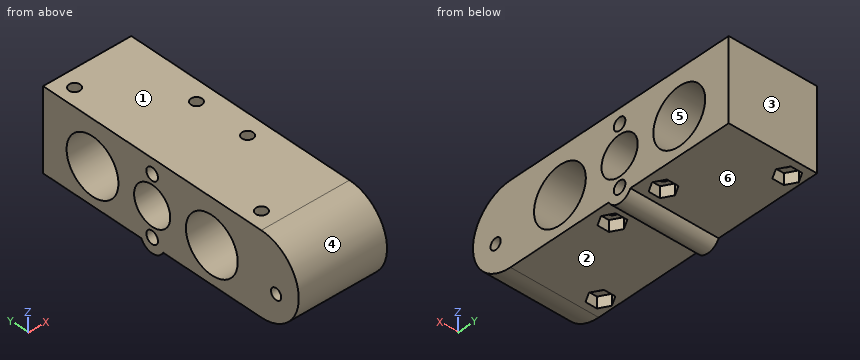
```python
from build123d import *

# Parameters (mm, degrees)
SKETCH035_R          = 7.6
SKETCH035_R_2        = 1.5
PAD011_DEPTH         = 24
SKETCH034_R          = 5.3
SKETCH034_R_2        = 1.7
POCKET021_DEPTH      = 24.001
SKETCH036_R          = 1.5
POCKET022_DEPTH      = 22.001
POCKET022_DEPTH_BACK = 2.001
POCKET023_DEPTH      = 3


with BuildPart() as part:
    # Sketch035 → Pad011 (new body)
    with BuildSketch(Plane.YZ):
        with BuildLine():
            Line((-32, 12), (32, 12))
            Line((32, 12), (32, -10))
            Line((3.1622776602, -10), (32, -10))
            ThreePointArc((-3.1622776602, -10), (0, -12), (3.1622776602, -10))
            Line((-32, -10), (-3.1622776602, -10))
            ThreePointArc((-32, 12), (-43, 1), (-32, -10))
        make_face()
        with Locations((17.5, 0)):
            Circle(SKETCH035_R, mode=Mode.SUBTRACT)
        with Locations((-17.5, 0)):
            Circle(SKETCH035_R, mode=Mode.SUBTRACT)
        with Locations((-36.35, -1.62)):
            Circle(SKETCH035_R_2, mode=Mode.SUBTRACT)
    extrude(amount=PAD011_DEPTH)

    # Sketch034 → Pocket021 (cut, through all)
    with BuildSketch(Plane(origin=(0, 0, 0), x_dir=(0, 0.7071067812, 0.7071067812), z_dir=(1, 0, 0))):
        Circle(SKETCH034_R)
        with Locations((5.65, 5.65)):
            Circle(SKETCH034_R_2)
        with Locations((-5.65, -5.65)):
            Circle(SKETCH034_R_2)
    extrude(amount=POCKET021_DEPTH, mode=Mode.SUBTRACT)

    # Sketch036 (on DatumPlane) → Pocket022 (cut, two sides)
    with BuildSketch(Plane.YX.offset(10)) as pocket022_sk:
        with Locations((-7.5, 19)):
            Circle(SKETCH036_R)
        with Locations((7.5, 19)):
            Circle(SKETCH036_R)
        with Locations((27.4, 4.3)):
            Circle(SKETCH036_R)
        with Locations((-27.4, 4.3)):
            Circle(SKETCH036_R)
    extrude(amount=-POCKET022_DEPTH, mode=Mode.SUBTRACT)
    extrude(pocket022_sk.sketch, amount=POCKET022_DEPTH_BACK, mode=Mode.SUBTRACT)

    # Sketch037 (on DatumPlane) → Pocket023 (cut)
    with BuildSketch(Plane.YX.offset(10)):
        Polygon((-24.7, 5.3588457268), (-27.4, 6.9176914536), (-30.1, 5.3588457268), (-30.1, 2.2411542732), (-27.4, 0.6823085464), (-24.7, 2.2411542732), align=None)
        Polygon((24.7, 5.3588457268), (24.7, 2.2411542732), (27.4, 0.6823085464), (30.1, 2.2411542732), (30.1, 5.3588457268), (27.4, 6.9176914536), align=None)
        Polygon((10.2, 20.5588457268), (7.5, 22.1176914536), (4.8, 20.5588457268), (4.8, 17.4411542732), (7.5, 15.8823085464), (10.2, 17.4411542732), align=None)
        Polygon((-7.5, 22.1176914536), (-10.2, 20.5588457268), (-10.2, 17.4411542732), (-7.5, 15.8823085464), (-4.8, 17.4411542732), (-4.8, 20.5588457268), align=None)
    extrude(amount=-POCKET023_DEPTH, mode=Mode.SUBTRACT)


with BuildPart() as part_1:
    # Body006 placement: moved
    add(part.part.moved(Location((0, 0, -50))))


solid = part_1.part
```
Work out the finished part from the listing and answer in its coordinate system (mm). Face numbers are marked on the shaded views. A direction names the side the tool comes from. Give positions to 0.01 mm unless a question says otherwise; leave off trailing zeros. Order: outer loops, then holes, each group sorted by start corner. A loop starts at its lowest first (then second) coordinate and runs counter-clockwise, first axis right, second up. Notation, with made-up numbers: M 36.25,66.5 L 53.25,66.5 A28 cw 53.25,96.5 Z; hole C -39.75,25 d9. An arc over 180 degrees is marked long. Return JSON: item names as keys, results as strings.
1) Straight lines are drawn through the part: line 1 along Z through (x, y) = (5.75, -17.5); line 2 along Y through (x, z) = (5.25, -45.5); line 3 along Y through (x, z) = (20.25, -54.75). For each, find the intervals that lie inside material, in ascending order. Write a range as [from, to].
Resolved:
{"line 1": "[-60, -57.6], [-42.4, -38]", "line 2": "[-42.43, -28.56], [-26.24, -23.62], [-11.38, -2.8], [2.8, 11.38], [23.62, 26.24], [28.56, 32]", "line 3": "[-41.38, -23.43], [-11.57, -8.33], [-6.67, -2.35], [2.35, 6.67], [8.33, 11.57], [23.43, 32]"}
2) Section C-C, the plane z = -48 is taken. Write down the section's boundary in (x, y).
Resolved:
{"outline": "M 0,-42.95 L 24,-42.95 L 24,-24.83 L 0,-24.83 Z; M 0,-10.17 L 24,-10.17 L 24,-4.91 L 0,-4.91 Z; M 0,4.91 L 24,4.91 L 24,10.17 L 0,10.17 Z; M 0,24.83 L 24,24.83 L 24,32 L 0,32 Z; hole C 4.3,-27.4 d3; hole C 4.3,27.4 d3; hole C 19,-7.5 d3; hole C 19,7.5 d3"}
3) A tool of negligible diameter and unlimited length cuts with its end or side. For the marked faces 1 and 2, from which of +Z, -Z, +X, -X, +Y, -Y can it reach the whole face along a straight path? Write none if from no direction.
Resolved:
{"face 1": "+Z, +X, -X, +Y, -Y", "face 2": "-Z, +X, -X, -Y"}
4) Each of these flat-tipped pins is pushed along its axis until it touches: pin 1 (12 mm diameter, centred on x = 11.5, y = -33.5, fed in from -Z); pin 2 (1.5 mm diameter, centred on x = 3, z = -58, fed in from -Y); pin 3 (1.6 mm diameter, centred on x = 19, y = -8.5, fed in from -Z). Where does it stop, or does it pass through?
Resolved:
{"pin 1": "z = -60", "pin 2": "y = -39.28", "pin 3": "z = -57"}
5) For a pull along Z with two mould halves and no side action, classify the marked faces 3, 4, 5 and 6 as +Z half, -Z half, draft (parallel to the pull), parting line (faces both ways), or undercut.
Resolved:
{"face 3": "draft", "face 4": "parting line", "face 5": "undercut", "face 6": "-Z half"}
6) Section B-B, the plane z = -51.62 is taken. Give the number of separate pieces and of enclosed holes in the cut face, plus the area to 3 significant figures.
Resolved:
{"separate pieces": "5", "enclosed holes": "4", "area": "737 mm^2"}
7) Section A-A, the plane y = 0 is taken. Write down the section's boundary in (x, z), plus the area to 3 significant figures.
Resolved:
{"outline": "M 0,-62 L 24,-62 L 24,-59.69 L 0,-59.69 Z; M 0,-56.29 L 24,-56.29 L 24,-55.3 L 0,-55.3 Z; M 0,-44.7 L 24,-44.7 L 24,-43.71 L 0,-43.71 Z; M 0,-40.31 L 24,-40.31 L 24,-38 L 0,-38 Z", "area": "158 mm^2"}
8) Section D-D, the plane y = -21 is taken. Write down the section's boundary in (x, z), plus the area to 3 significant figures.
Resolved:
{"outline": "M 0,-60 L 24,-60 L 24,-56.75 L 0,-56.75 Z; M 0,-43.25 L 24,-43.25 L 24,-38 L 0,-38 Z", "area": "204 mm^2"}
